from build123d import *

# Parameters (mm, degrees)
BOSS_EXTRUDE2_DEPTH = 38
BOSS_EXTRUDE3_DEPTH = 6
SKETCH6_R           = 6
SKETCH6_R_2         = 3
CUT_EXTRUDE1_DEPTH  = 91.111042609


with BuildPart() as part:
    # Sketch1 → Boss-Extrude2 (new body)
    with BuildSketch(Plane.XY):
        Polygon((52, 26), (24, 26), (24, 6), (0, 6), (0, 0), (17, 0), (17, -4), (22, 0), (54, 0), (59, -4), (59, 0), (76, 0), (76, 6), (52, 6), align=None)
    extrude(amount=BOSS_EXTRUDE2_DEPTH)

    # Sketch1_4 → Boss-Extrude3 (add)
    with BuildSketch(Plane.XY):
        Polygon((52, 6), (52, 26), (76, 6), align=None)
        Polygon((0, 6), (24, 6), (24, 26), align=None)
    extrude(amount=BOSS_EXTRUDE3_DEPTH)

    # Sketch6 → Cut-Extrude1 (cut, through all)
    with BuildSketch(Plane(origin=(0, 26, 0), x_dir=(1, 0, 0), z_dir=(0, 1, 0))):
        with Locations(Location((38, -16, 0), (0, 0, 270))):
            Circle(SKETCH6_R)
        with Locations(Location((65, -19, 0), (0, 0, 270))):
            Circle(SKETCH6_R_2)
        with Locations(Location((11, -19, 0), (0, 0, 270))):
            Circle(SKETCH6_R_2)
    extrude(amount=-CUT_EXTRUDE1_DEPTH, mode=Mode.SUBTRACT)


solid = part.part
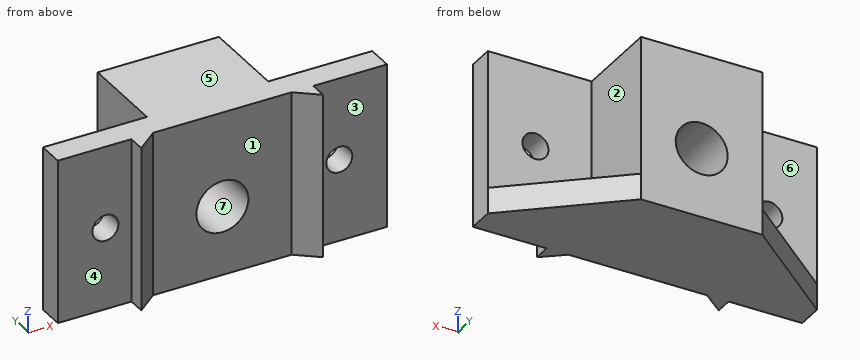
For this review, take the finished solid that the model builds, in its own axes (mm). Face numbers are marked on the shaded views. A direction names the side the tool comes from. Round coordinates to 2 decimals unless told otherwise and drop trailing zeros. Order: outer loops, then holes, each group sorted by start corner. A loop starts at its lowest first (then second) coordinate and runs counter-clockwise, first axis right, second up. Notation, with made-up numbers: M 22.25,-21 L 38.25,-21 A24 ccw 38.25,6 Z; hole C -13.75,44.5 d8. An arc over 180 degrees is marked long. Use a Markdown table: item, result. Add a question column.
Item 1: Tool access review of the marked faces 1, 2, 3 and 4: name each direction out of +Z, -Z, +X, -X, +Y, -Y from which nothing blocks a thin tool from reaching the whole face with its end or side.
Item 2: Add section D-D, the plane z = 19. Give the boundary of the cut face in (x, y).
Item 3: Mouldability with a two-part tool opening along Z and no side actions: class the marked faces 5, 6 and 7 as released by +Z, released by -Z, zero draft, split by the parting line, or undercut.
Item 4: Add section C-C, the plane z = 14.5. Give the boundary of the cut face in (x, y), then the cut area to 3 significant figures.
Item 5: To check wall thickness, follow line 1 along X through (y, z) = (17.5, 16); line 2 along Y through (x, z) = (25, 4); line 3 along Y through (x, z) = (54, 36.5). State the ranges of each line that lie inside material, in increasing order.
Item 6: Add section B-B, the plane y = 12. Give the boundary of the cut face in (x, z), then the cut area to 3 significant figures.
Item 7: Insertion check: pin 1 (1.2 mm diameter, centred on y = -2.5, z = 11, fed in from -X); pin 2 (12 mm diameter, centred on x = 8.5, z = 20.5, fed in from +Y); pin 3 (9.5 mm diameter, centred on x = 41, z = 9.5, fed in from -Y). Each pin has a flat end and moves straight along its axis. Give the tip position at first contact, or say it passes through.
Item 8: Add section A-A, the plane x = 38. Give the boundary of the cut face in (y, z).
Geometry results:
| question | item | result |
|---|---|---|
| 1 | face 1 | +Z, -Z, -Y |
| 1 | face 2 | +Z, +X, +Y |
| 1 | face 3 | +Z, -Z, +X, -Y |
| 1 | face 4 | +Z, -Z, -X, -Y |
| 2 | outline | M 0,0 L 8,0 L 8,6 L 0,6 Z; M 14,0 L 17,0 L 17,-4 L 22,0 L 32.8,0 L 32.8,26 L 24,26 L 24,6 L 14,6 Z; M 43.2,0 L 54,0 L 59,-4 L 59,0 L 62,0 L 62,6 L 52,6 L 52,26 L 43.2,26 Z; M 68,0 L 76,0 L 76,6 L 68,6 Z |
| 3 | face 5 | released by +Z |
| 3 | face 6 | zero draft |
| 3 | face 7 | undercut |
| 4 | outline | M 0,0 L 17,0 L 17,-4 L 22,0 L 32.19,0 L 32.19,26 L 24,26 L 24,6 L 0,6 Z; M 43.81,0 L 54,0 L 59,-4 L 59,0 L 76,0 L 76,6 L 52,6 L 52,26 L 43.81,26 Z |
| 4 | area | 734 mm² |
| 5 | line 1 | x = 24 to 32, 44 to 52 |
| 5 | line 2 | y = 0 to 26 |
| 5 | line 3 | y = 0 to 6 |
| 6 | outline | M 7.2,0 L 68.8,0 L 68.8,6 L 52,6 L 52,38 L 24,38 L 24,6 L 7.2,6 Z; hole C 38,16 d12 |
| 6 | area | 1,150 mm² |
| 7 | pin 1 | stops at x = 17 |
| 7 | pin 2 | stops at y = 6 |
| 7 | pin 3 | stops at y = 0 |
| 8 | outline | M 0,0 L 26,0 L 26,10 L 0,10 Z; M 0,22 L 26,22 L 26,38 L 0,38 Z |
